Autodesk Inventor part; units mm, degrees
ref_plane "YZ Plane" through (0, 0, 0) normal (1, 0, 0) x (0, 1, 0)
ref_plane "XZ Plane" through (0, 0, 0) normal (0, 1, 0) x (-1, 0, 0)
ref_plane "XY Plane" through (0, 0, 0) normal (0, 0, 1) x (1, 0, 0)
sketch "Эскиз1" plane through (0, 0, 0) normal (0, 1, 0) x (-1, 0, 0)
  line L0 (21, 30) -> (-21, 30)
  line L1 (-21, 30) -> (-21, -30)
  line L2 (-21, -30) -> (21, -30)
  line L3 (21, -30) -> (21, 30)
  line L4 (21, 30) -> (-21, -30) construction
  line L5 (-21, 30) -> (21, -30) construction
  point P0 (0, 0)
  dimension "d0" = 42
  dimension "d1" = 60
extrude "Выдавливание1" add sketch "Эскиз1" along normal blind 4
sketch "Эскиз4" plane through (0, 4, 0) normal (0, 1, 0) x (1, 0, 0)
  circle A0 centre (-13, -24) radius 1.6
  circle A1 centre (12.5, -24) radius 1.6
  circle A2 centre (12.5, 24) radius 1.6
  circle A3 centre (-13, 24) radius 1.6
  line L0 (-21, 30) -> (-21, -30)
  line L1 (-21, -30) -> (21, -30)
  line L2 (21, -30) -> (21, 30)
  line L3 (21, 30) -> (-21, 30)
  point P0 (0, 0)
  dimension "d28" = 3.2
  dimension "d29" = 3.2
  dimension "d31" = 3.2
  dimension "d32" = 8
  dimension "d33" = 6
  dimension "d34" = 6
  dimension "d36" = 6
  dimension "d37" = 6
  dimension "d38" = 8
  dimension "d56" = 25.5
  dimension "d57" = 3.2
  dimension "d58" = 25.5
extrude "Выдавливание3" cut sketch "Эскиз4" against normal blind 10 contours A0 | A1 | A2 | A3
sketch "Эскиз5" plane through (0, 4, 0) normal (0, 1, 0) x (1, 0, 0)
  line L0 (21, -30) -> (21, 30)
  line L1 (21, -8.3) -> (11, -8.3)
  line L2 (11, -8.3) -> (11, -11.7)
  line L3 (11, -11.7) -> (21, -11.7)
  line L4 (21, -11.7) -> (21, -8.3)
  line L5 (21, 8.3) -> (11, 8.3)
  line L6 (11, 8.3) -> (11, 11.7)
  line L7 (11, 11.7) -> (21, 11.7)
  line L8 (21, 11.7) -> (21, 8.3)
  line L9 (0, 0) -> (21, 0) construction
  line L10 (15.5, -7.25) -> (13.2, -7.25)
  line L11 (13.2, -7.25) -> (13.2, -12.75)
  line L12 (13.2, -12.75) -> (15.5, -12.75)
  line L13 (15.5, -12.75) -> (15.5, -7.25)
  line L14 (15.5, -7.25) -> (13.2, -12.75) construction
  line L15 (13.2, -7.25) -> (15.5, -12.75) construction
  line L16 (13.2, 7.25) -> (15.5, 7.25)
  line L17 (15.5, 7.25) -> (15.5, 12.75)
  line L18 (15.5, 12.75) -> (13.2, 12.75)
  line L19 (13.2, 12.75) -> (13.2, 7.25)
  line L20 (13.2, 7.25) -> (15.5, 12.75) construction
  line L21 (15.5, 7.25) -> (13.2, 12.75) construction
  point P0 (21, -10)
  point P1 (21, 10)
  point P2 (14.35, -10)
  point P3 (14.35, 10)
  point P4 (15.5, -10)
  point P5 (15.5, -11.7)
  point P6 (21, -11.7)
  point P7 (15.5, -8.3)
  point P8 (13.2, -8.3)
  point P9 (13.2, -11.7)
  point P10 (13.2, 8.3)
  point P11 (15.5, 8.3)
  point P12 (21, 8.3)
  point P13 (21, 11.7)
  point P14 (15.5, 11.7)
  point P15 (13.2, 11.7)
  dimension "d42" = 10
  dimension "d43" = 3.4
  dimension "d44" = 10
  dimension "d45" = 3.4
  dimension "d46" = 10
  dimension "d47" = 10
  dimension "d48" = 2.3
  dimension "d49" = 5.5
  dimension "d50" = 2.3
  dimension "d51" = 5.5
  dimension "d52" = 5.5
  dimension "d53" = 5.5
extrude "Выдавливание4" cut sketch "Эскиз5" against normal blind 4
properties part number "каретки_потолок"
Design review of the part built by this model. Coordinates are the model's own, in mm. A direction names the side the tool comes from. Give positions to 0.01 mm unless a question says otherwise; leave off trailing zeros. Order: outer loops, then holes, each group sorted by start corner. A loop starts at its lowest first (then second) coordinate and runs counter-clockwise, first axis right, second up. Notation, with made-up numbers: (-16, -6.5) - (25, -6.5) arc R18 ccw to (25, 19.5) - close; hole circle Ø11 at (15.5, -33.5). An arc over 180 degrees is marked (long way). Write item = value, one per line. Start each with the question number.
Q1. Tool access review of faces 5 (the face through (14, 2, -12.75)), 6 (the face through (18, 2, 8.3)), 7 (the face through (21, 2, 0)): name each direction out of +Z, -Z, +X, -X, +Y, -Y from which nothing blocks a thin tool from reaching the whole face with its end or side.
Q2. We need section D-D on x = -13. State the section outline as (y, z) points.
Q3. We need section C-C on y = 1.15. State how many separate pieces and enclosed holes the cut face has, plus the area to 3 significant figures.
Q4. To check wall thickness, follow L1, parallel to X at y = 2.8, z = 24; L2, parallel to Z at x = 12.5, y = 2.65; L3, parallel to Z at x = 15, y = 2.9. State the ranges of each line that lie inside material, in increasing order. Write a range as from..to.
Q5. We need section A-A on x = 12.5. State the section outline as (y, z) points, plus the area to 3 significant figures.
Q6. Mouldability with a two-part tool opening along Z and no side actions: class faces 1 (the face through (18, 2, 11.7)), 2 (the face through (12, 2, 8.3)), 3 (the face through (0, 4, 0)), 4 (the face through (0, 2, 30)) as released by +Z, released by -Z, zero draft, split by the parting line, or undercut.
Q7. We need section B-B on z = 24. State the section outline as (x, y) points.
Working result:
q1.face_5 = +Y, -Y
q1.face_6 = +X, +Y, -Y
q1.face_7 = +Z, -Z, +X, +Y, -Y
q2.outline = (0, -30) - (4, -30) - (4, -25.6) - (0, -25.6) - close; (0, -22.4) - (4, -22.4) - (4, 22.4) - (0, 22.4) - close; (0, 25.6) - (4, 25.6) - (4, 30) - (0, 30) - close
q3.separate_pieces = 1
q3.enclosed_holes = 4
q3.area = 2,410 mm²
q4.L1 = -21..-14.6, -11.4..10.9, 14.1..21
q4.L2 = -30..-25.6, -22.4..-11.7, -8.3..8.3, 11.7..22.4, 25.6..30
q4.L3 = -30..-12.75, -7.25..7.25, 12.75..30
q5.outline = (0, -30) - (4, -30) - (4, -25.6) - (0, -25.6) - close; (0, -22.4) - (4, -22.4) - (4, -11.7) - (0, -11.7) - close; (0, -8.3) - (4, -8.3) - (4, 8.3) - (0, 8.3) - close; (0, 11.7) - (4, 11.7) - (4, 22.4) - (0, 22.4) - close; (0, 25.6) - (4, 25.6) - (4, 30) - (0, 30) - close
q5.area = 187 mm²
q6.face_1 = undercut
q6.face_2 = undercut
q6.face_3 = zero draft
q6.face_4 = released by +Z
q7.outline = (-21, 0) - (-14.6, 0) - (-14.6, 4) - (-21, 4) - close; (-11.4, 0) - (10.9, 0) - (10.9, 4) - (-11.4, 4) - close; (14.1, 0) - (21, 0) - (21, 4) - (14.1, 4) - close
